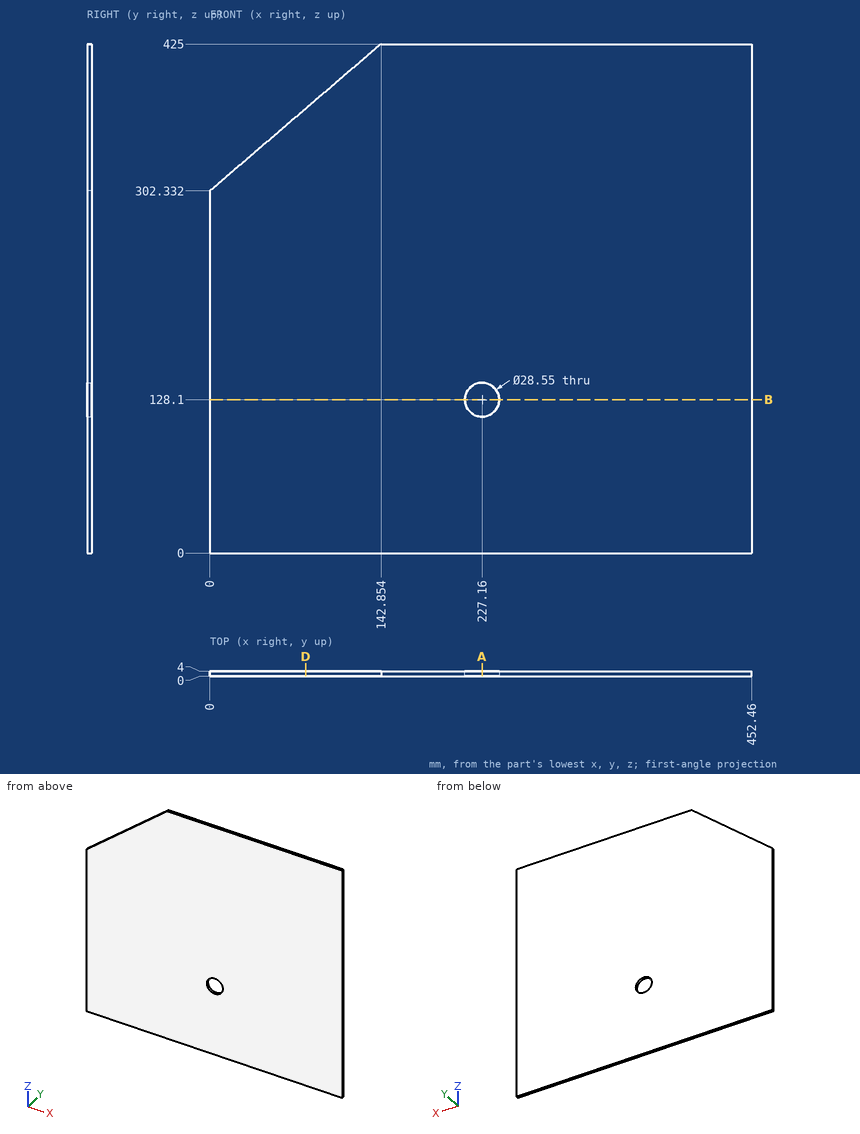
Study the drawing (mm; zero at the part's minimum x, y, z) and answer. Coordinates: 2 decimals unless noted, no trailing zeros. Write each loop counter-clockwise with the first axis right and the second up, starting at its lowest first coordinate (ties: lowest second). Pieces come first, ordered by that corner, then holes.
Q1. Section A-A, the plane x = 227.16 is taken. Write down the section's boundary in (y, z) (1 decimal).
Returned:
outline: (0, 0) - (4, 0) - (4, 113.8) - (0, 113.8) - close; (0, 142.4) - (4, 142.4) - (4, 425) - (0, 425) - close
Q2. Section B-B, the plane z = 128.1 is taken. Write down the section's boundary in (x, y) (1 decimal).
Returned:
outline: (0, 0) - (212.9, 0) - (212.9, 4) - (0, 4) - close; (241.4, 0) - (452.5, 0) - (452.5, 4) - (241.4, 4) - close
Q3. Section D-D, the plane x = 80 is taken. Write down the section's boundary in (y, z).
Returned:
outline: (0, 0) - (4, 0) - (4, 371.03) - (0, 371.03) - close
Q4. Find the intervals of material crossed by line 1 along X through (y, z) = (3, 128.1) (1 decimal); line 2 along Z through (x, y) = (227.16, 1.4) (1 decimal); line 3 along Z through (x, y) = (120, 0.3) (1 decimal), in increasing order.
Returned:
line 1: x = 0 to 212.9, 241.4 to 452.5
line 2: z = 0 to 113.8, 142.4 to 425
line 3: z = 0 to 405.4
Q5. Given P1, Ø1.5, axis at y = 1.5, z = 325.5, coming from the -X side (1 decimal), flat-ended and moving along its own axis, determine where the tip first touches the part or whether it passes through.
Returned:
P1: stops at x = 26.1
